Model file for the job. Use its own axes, mm. Round coordinates to 2 decimals unless told otherwise and drop trailing zeros. Write item = value, one per line.
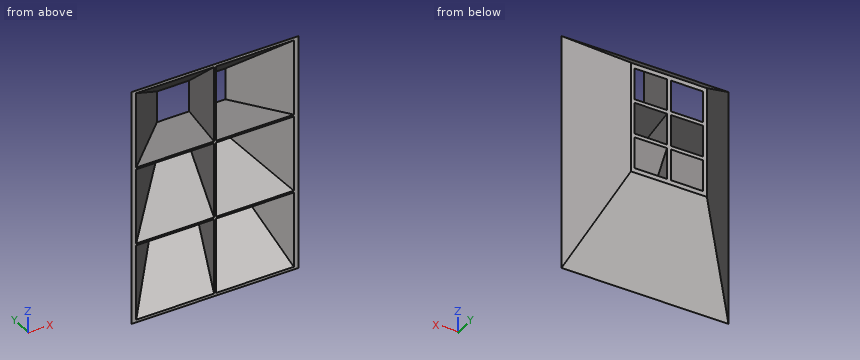
```python
from build123d import *

# Parameters (mm, degrees)
EXTRUDE_1_DEPTH          = 64
CUT_EXTRUDE_1_DEPTH      = 18.501606075
CUT_EXTRUDE_1_DEPTH_BACK = 27.498393925
SKETCH_4_W               = 8.5
SKETCH_4_H               = 8.5
SKETCH_3_W               = 20.5
SKETCH_3_H               = 20.5
SKETCH_4_3_W             = 8.5
SKETCH_4_3_H             = 8.5
SKETCH_3_3_W             = 20.5
SKETCH_3_3_H             = 20.5
SKETCH_4_4_W             = 8.5
SKETCH_4_4_H             = 8.5
SKETCH_3_4_W             = 20.5
SKETCH_3_4_H             = 20.5
SKETCH_4_5_W             = 8.5
SKETCH_4_5_H             = 8.5
SKETCH_3_5_W             = 20.5
SKETCH_3_5_H             = 20.5
SKETCH_4_6_W             = 8.5
SKETCH_4_6_H             = 8.5
SKETCH_3_6_W             = 20.5
SKETCH_3_6_H             = 20.5
SKETCH_4_7_W             = 8.5
SKETCH_4_7_H             = 8.5
SKETCH_3_7_W             = 20.5
SKETCH_3_7_H             = 20.5


with BuildPart() as part:
    # Sketch 1 → Extrude 1 (new body)
    with BuildSketch(Plane.XY):
        Polygon((0, 0), (44, 0), (37.501606075, 20), (17.501606075, 20), align=None)
    extrude(amount=EXTRUDE_1_DEPTH)

    # Sketch 2 → Cut-Extrude 1 (cut, two sides)
    with BuildSketch(Plane.ZY.offset(-17.501606075)) as cut_extrude_1_sk:
        Polygon((0, 0), (17, 20), (0, 20), align=None)
        Polygon((64, 0), (47, 20), (64, 20), align=None)
    extrude(amount=CUT_EXTRUDE_1_DEPTH, mode=Mode.SUBTRACT)
    extrude(cut_extrude_1_sk.sketch, amount=-CUT_EXTRUDE_1_DEPTH_BACK, mode=Mode.SUBTRACT)

    # Sketch 4 → Loft 1 section 0
    with BuildSketch(Plane(origin=(0, 20, 0), x_dir=(1, 0, 0), z_dir=(0, 1, 0))):
        with Locations((22.751606075, -22.5)):
            Rectangle(SKETCH_4_W, SKETCH_4_H)
    # Sketch 3 → Loft 1 section 1
    with BuildSketch(Plane.XZ):
        with Locations((11.5, 11)):
            Rectangle(SKETCH_3_W, SKETCH_3_H)
    loft(mode=Mode.SUBTRACT)

    # Sketch 4_3 → Loft 2 section 0
    with BuildSketch(Plane(origin=(0, 20, 0), x_dir=(1, 0, 0), z_dir=(0, 1, 0))):
        with Locations((22.751606075, -32)):
            Rectangle(SKETCH_4_3_W, SKETCH_4_3_H)
    # Sketch 3_3 → Loft 2 section 1
    with BuildSketch(Plane.XZ):
        with Locations((11.5, 32)):
            Rectangle(SKETCH_3_3_W, SKETCH_3_3_H)
    loft(mode=Mode.SUBTRACT)

    # Sketch 4_4 → Loft 3 section 0
    with BuildSketch(Plane(origin=(0, 20, 0), x_dir=(1, 0, 0), z_dir=(0, 1, 0))):
        with Locations((22.751606075, -41.5)):
            Rectangle(SKETCH_4_4_W, SKETCH_4_4_H)
    # Sketch 3_4 → Loft 3 section 1
    with BuildSketch(Plane.XZ):
        with Locations((11.5, 53)):
            Rectangle(SKETCH_3_4_W, SKETCH_3_4_H)
    loft(mode=Mode.SUBTRACT)

    # Sketch 4_5 → Loft 4 section 0
    with BuildSketch(Plane(origin=(0, 20, 0), x_dir=(1, 0, 0), z_dir=(0, 1, 0))):
        with Locations((32.251606075, -22.5)):
            Rectangle(SKETCH_4_5_W, SKETCH_4_5_H)
    # Sketch 3_5 → Loft 4 section 1
    with BuildSketch(Plane.XZ):
        with Locations((32.5, 11)):
            Rectangle(SKETCH_3_5_W, SKETCH_3_5_H)
    loft(mode=Mode.SUBTRACT)

    # Sketch 4_6 → Loft 5 section 0
    with BuildSketch(Plane(origin=(0, 20, 0), x_dir=(1, 0, 0), z_dir=(0, 1, 0))):
        with Locations((32.251606075, -32)):
            Rectangle(SKETCH_4_6_W, SKETCH_4_6_H)
    # Sketch 3_6 → Loft 5 section 1
    with BuildSketch(Plane.XZ):
        with Locations((32.5, 32)):
            Rectangle(SKETCH_3_6_W, SKETCH_3_6_H)
    loft(mode=Mode.SUBTRACT)

    # Sketch 4_7 → Loft 6 section 0
    with BuildSketch(Plane(origin=(0, 20, 0), x_dir=(1, 0, 0), z_dir=(0, 1, 0))):
        with Locations((32.251606075, -41.5)):
            Rectangle(SKETCH_4_7_W, SKETCH_4_7_H)
    # Sketch 3_7 → Loft 6 section 1
    with BuildSketch(Plane.XZ):
        with Locations((32.5, 53)):
            Rectangle(SKETCH_3_7_W, SKETCH_3_7_H)
    loft(mode=Mode.SUBTRACT)


solid = part.part
```
1) Flat gauge pins, fed straight in: pin 1 Ø1 at (y, z) = (4.5, 52.5) entering from -X; pin 2 Ø6 at (x, y) = (23, 12.5) entering from +Z (3 decimals); pin 3 Ø4 at (x, y) = (19, 6) entering from -Z. Where does each tip first touch, or does it go through?
Conclusion:
pin_1 = 3.5
pin_2 = 55.925
pin_3 = 3.4
2) Wall check: line 1 along Z through (x, y) = (21, 17.75) (1 decimal); line 2 along X through (y, z) = (7.5, 29.5); line 3 along X through (y, z) = (5.75, 45). Give the ranges that are in metal, low to high.
Conclusion:
line_1 = 15.1 to 16.3, 26.1 to 27.1, 36.9 to 37.9, 47.7 to 48.9
line_2 = 6.56 to 7.72, 23.72 to 24.41, 40.41 to 41.56
line_3 = 5.03 to 6.21, 23.26 to 23.9, 40.95 to 42.13
3) Cut at A-A (z = 44.5). Give the number of separate pieces and of enclosed holes in the cut face, and give its area (3 significant figures).
Conclusion:
separate_pieces = 3
enclosed_holes = 0
area = 60.0 mm^2
